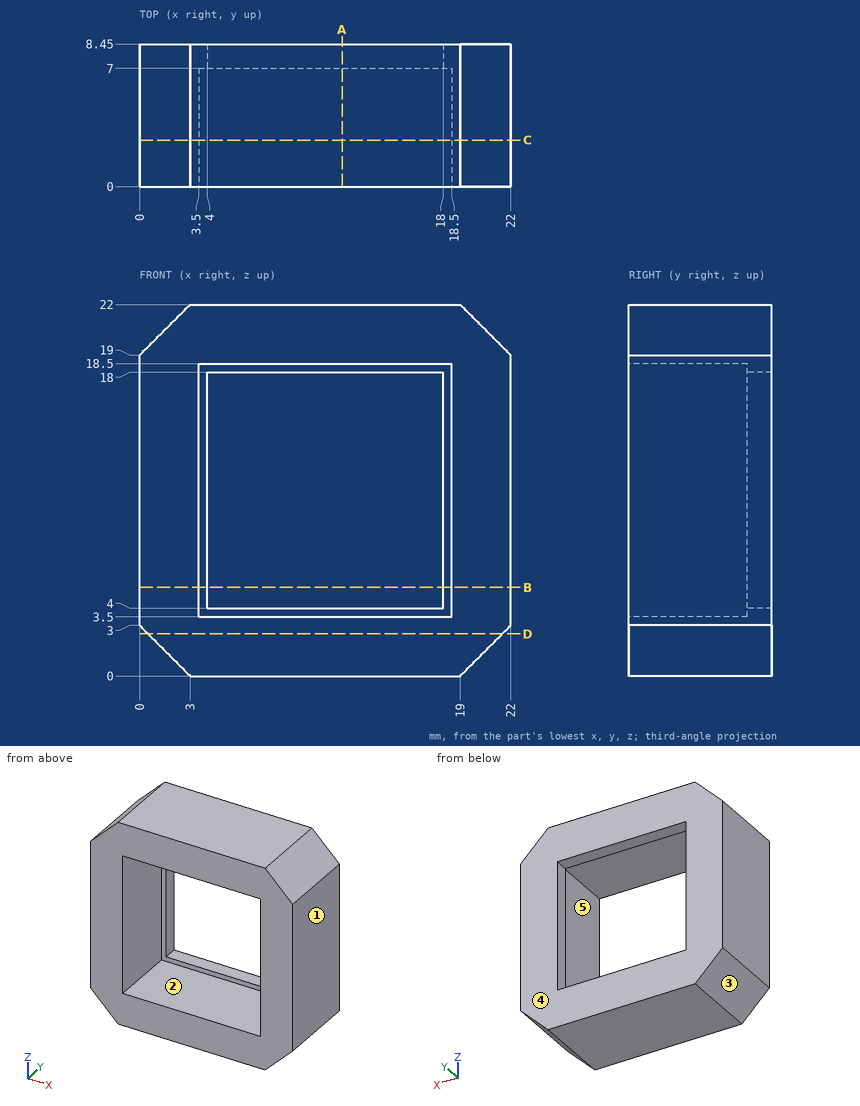
Verification items for this drawing (mm, ordinates from the low corner). A direction names the side the tool comes from. Give positions to 0.01 mm unless a question says otherwise; leave off trailing zeros. Loops run counter-clockwise (first coordinate to the right, second up) from the corner with the lowest first, then second, coordinate; pieces in that order, holes last. Notation, with made-up numbers: M 19,67 L 62,67 A10 ccw 62,73 Z; hole C 71,31.5 d5. An arc over 180 degrees is marked long. Answer in a Markdown table with one row per item.
1) Mould release check, pull along Z, two halves, no side actions. Record for the marked faces 1, 2 and 3: released by +Z, released by -Z, zero draft, split by the parting line, or undercut.
Solutions:
| item | result |
|---|---|
| face 1 | zero draft |
| face 2 | undercut |
| face 3 | released by -Z |
2) Tool access check on the marked faces 4 and 5. Record the directions out of +Z, -Z, +X, -X, +Y, -Y that give a thin tool (end or side, any length) a straight path to the whole face; none if there is none.
Solutions:
| item | result |
|---|---|
| face 4 | +Z, -Z, +X, -X, +Y |
| face 5 | -Y |
3) Depth check by flat-ended pin: pin 1 (7.5 mm diameter, centred on x = 14, z = 7.5, fed in from -Y). Enter the tip coordinate at first touch or a pass-through.
Solutions:
| item | result |
|---|---|
| pin 1 | stops at y = 7 |
4) Cross-section at B-B (z = 5.25). Enter the section's corners in (x, y).
Solutions:
| item | result |
|---|---|
| outline | M 0,0 L 3.5,0 L 3.5,7 L 4,7 L 4,8.45 L 0,8.45 Z; M 18,7 L 18.5,7 L 18.5,0 L 22,0 L 22,8.45 L 18,8.45 Z |
5) Thickness scan on line 1 (Z direction, x = 5, y = 2); line 2 (X direction, y = 7.25, z = 12.25). Record the ranges inside material, lowest first.
Solutions:
| item | result |
|---|---|
| line 1 | z = 0 to 3.5, 18.5 to 22 |
| line 2 | x = 0 to 4, 18 to 22 |
6) Cross-section at C-C (y = 2.75). Enter the section's corners in (x, z), plus the area to 3 significant figures.
Solutions:
| item | result |
|---|---|
| outline | M 0,3 L 3,0 L 19,0 L 22,3 L 22,19 L 19,22 L 3,22 L 0,19 Z; hole M 3.5,3.5 L 18.5,3.5 L 18.5,18.5 L 3.5,18.5 Z |
| area | 241 mm^2 |
7) Cross-section at A-A (x = 12). Enter the section's corners in (y, z), plus the area to 3 significant figures.
Solutions:
| item | result |
|---|---|
| outline | M 0,0 L 8.45,0 L 8.45,4 L 7,4 L 7,3.5 L 0,3.5 Z; M 0,18.5 L 7,18.5 L 7,18 L 8.45,18 L 8.45,22 L 0,22 Z |
| area | 60.6 mm^2 |
8) Cross-section at D-D (z = 2.5). Enter the section's corners in (x, y), plus the area to 3 significant figures.
Solutions:
| item | result |
|---|---|
| outline | M 0.5,0 L 21.5,0 L 21.5,8.45 L 0.5,8.45 Z |
| area | 177 mm^2 |
